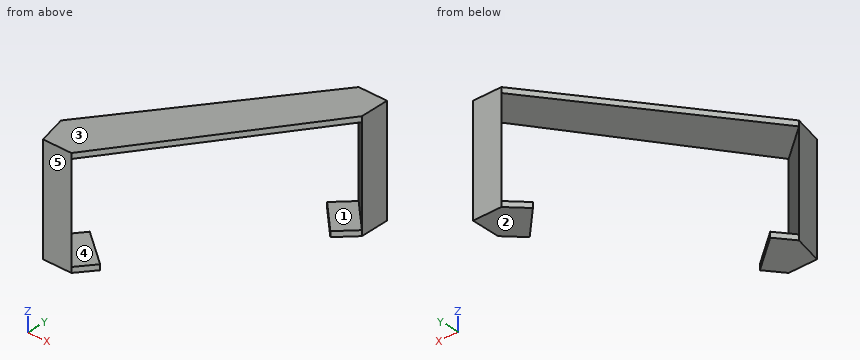
from build123d import *

# Parameters (mm, degrees)
BOSS_EXTRUDE1_DEPTH = 2
BOSS_EXTRUDE2_DEPTH = 38.1
BOSS_EXTRUDE3_DEPTH = 2


with BuildPart() as part:
    # Sketch1 → Boss-Extrude1 (new body)
    with BuildSketch(Plane.XY):
        Polygon((29.528587169, 36.011013454), (-21.569396066, -32.119630858), (-18.916193719, -42.719630858), (-8.306193719, -42.719630858), (40.131789515, 25.401013454), (40.131789515, 36.011013454), align=None)
    extrude(amount=BOSS_EXTRUDE1_DEPTH)

    # Sketch2 → Boss-Extrude2 (add)
    with BuildSketch(Plane(origin=(0, 0, 0), x_dir=(-1, 0, 0), z_dir=(0, 0, -1))):
        Polygon((-40.131789515, 25.401013454), (-29.528587169, 36.011013454), (-40.131789515, 36.011013454), align=None)
        Polygon((8.306193719, -42.719630858), (21.569396066, -32.119630858), (18.916193719, -42.719630858), align=None)
    extrude(amount=BOSS_EXTRUDE2_DEPTH)

    # Sketch3 → Boss-Extrude3 (add)
    with BuildSketch(Plane(origin=(0, 0, -38.1), x_dir=(-1, 0, 0), z_dir=(0, 0, -1))):
        Polygon((21.569396066, -32.119630858), (8.306193719, -42.719630858), (3.194123868, -36.323176439), (16.457326214, -25.723176439), align=None)
        Polygon((-29.528587169, 36.011013454), (-40.131789515, 25.401013454), (-33.863813996, 19.137053724), (-23.260611649, 29.747053724), align=None)
    extrude(amount=-BOSS_EXTRUDE3_DEPTH)


solid = part.part
Geometry check sheet. Reference: the model listing, model coordinates, mm. Face numbers are marked on the shaded views. A direction names the side the tool comes from. Give positions to 0.01 mm unless a question says otherwise; leave off trailing zeros. Loops run counter-clockwise (first coordinate to the right, second up) from the corner with the lowest first, then second, coordinate; pieces in that order, holes last. Notation, with made-up numbers: (31.25, 67.25) -> (73.25, 67.25) arc R15 cw to (73.25, 93.25) -> close; hole circle Ø6 at (71, 87.5). An arc over 180 degrees is marked (long way). Answer in a Markdown table with one row per item. Add a question column.
1) Draft check along Z on the marked faces 1, 2 and 3. Enter one of: pulls with the +Z half, pulls with the -Z half, needs draft (parallel to the pull), parting line crosses it, or undercut.
2) Set-up check for the marked faces 4 and 5: record each of +Z, -Z, +X, -X, +Y, -Y from which the full face is reachable in a straight line by a thin tool's end or side.
3) Cross-section at D-D on x = 2.5. Record the boundary of the cut face in (y, z), and give its area (3 significant figures).
4) Cross-section at A-A on x = 26.5. Record the boundary of the cut face in (y, z).
5) Material ranges on probe 1 along Z at (x, y) = (0, -7.5); probe 2 along Y at (x, z) = (-13, -25.5); probe 3 along Y at (x, z) = (-17, -5), recorded low to high. Write a range as from..to.
6) Gauge pin test, flat ends, axial feed: P1, Ø3, axis at y = -29.5, z = -20.5, coming from the -X side; P2, Ø2, axis at x = 27, y = 20.5, coming from the -Z side; P3, Ø8, axis at x = 25, z = -3, coming from the +Y side. Record the tip position at first contact, or that the pin passes through.
7) Cross-section at C-C on y = 22.5. Record the boundary of the cut face in (x, z), and give its area (3 significant figures).
8) Cross-section at B-B on z = -7.5. Record the boundary of the cut face in (x, y).
Outcome:
| question | item | result |
|---|---|---|
| 1 | face 1 | undercut |
| 1 | face 2 | pulls with the -Z half |
| 1 | face 3 | pulls with the +Z half |
| 2 | face 4 | +X, +Y |
| 2 | face 5 | +Z, -Z, +X, -X, -Y |
| 3 | outline | (-27.52, 0) -> (-0.03, 0) -> (-0.03, 2) -> (-27.52, 2) -> close |
| 3 | area | 55.0 mm^2 |
| 4 | outline | (6.23, 0) -> (31.97, 0) -> (31.97, 2) -> (6.23, 2) -> close; (26.51, -38.1) -> (32.98, -38.1) -> (32.98, -36.1) -> (26.51, -36.1) -> close |
| 5 | probe 1 | z = 0..2 |
| 5 | probe 2 | y = -42.72..-38.97 |
| 5 | probe 3 | y = -42.72..-35.77 |
| 6 | P1 | passes through |
| 6 | P2 | stops at z = 0 |
| 6 | P3 | stops at y = 33.5 |
| 7 | outline | (19.4, 0) -> (38.07, 0) -> (38.07, 2) -> (19.4, 2) -> close; (30.5, -38.1) -> (37.23, -38.1) -> (37.23, -36.1) -> (30.5, -36.1) -> close |
| 7 | area | 50.8 mm^2 |
| 8 | outline | (-21.57, -32.12) -> (-18.92, -42.72) -> (-8.31, -42.72) -> close; (29.53, 36.01) -> (40.13, 25.4) -> (40.13, 36.01) -> close |
